from build123d import *

# Parameters (mm, degrees)
F0_R     = 8.5
F1_DEPTH = 18
F3_DEPTH = 11
F4_R     = 10
F5_DEPTH = 11
F7_DEPTH = 10


with BuildPart() as f1:
    # F0 (on Top) → F1 (new body)
    with BuildSketch(Plane.XY):
        Circle(F0_R)
        with BuildLine():
            ThreePointArc((-5.44875, -2.512196), (-5.196152, 3), (-0.54875, 5.974853))
            Line((-0.54875, 5.974853), (5.44875, 2.512196))
            ThreePointArc((5.44875, 2.512196), (5.196152, -3), (0.54875, -5.974853))
            Line((0.54875, -5.974853), (-5.44875, -2.512196))
        make_face(mode=Mode.SUBTRACT)
    extrude(amount=F1_DEPTH)

    # F2 (on Top) → F3 (join)
    with BuildSketch(Plane.XY):
        Polygon((0.509195, 6.881952), (-5.705348, -3.881952), (-0.509195, -6.881952), (0, -6), (5.705348, 3.881952), align=None)
    extrude(amount=F3_DEPTH)

    # F4 (on Top) → F5 (join)
    with BuildSketch(Plane.XY):
        Circle(F4_R)
    extrude(amount=-F5_DEPTH)

    # F6 (on face) → F7 (join)
    with BuildSketch(Plane(origin=(0, 0, -11), x_dir=(1, 0, 0), z_dir=(0, 0, -1))):
        with BuildLine():
            Line((3, -69.539392), (3, -9.539392))
            ThreePointArc((3, -9.539392), (0, 10), (-3, -9.539392))
            Line((-3, -9.539392), (-3, -69.539392))
            Line((-3, -69.539392), (3, -69.539392))
        make_face()
    extrude(amount=F7_DEPTH)


solid = f1.part
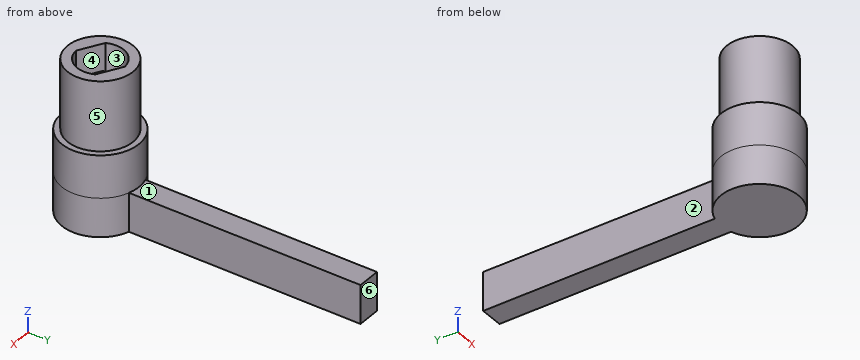
Design review of the part built by this model. Coordinates are the model's own, in mm. Face numbers are marked on the shaded views. A direction names the side the tool comes from. Coordinates: 2 decimals unless noted, no trailing zeros. Loops run counter-clockwise (first coordinate to the right, second up) from the corner with the lowest first, then second, coordinate; pieces in that order, holes last. Notation, with made-up numbers: M 5.25,-5 L 14.25,-5 A22 ccw 14.25,24 Z; hole C 60.25,45 d8. An arc over 180 degrees is marked long. Answer as CSV lines item,"result".
Item 1: The part is to be moulded in two halves that separate along Y. For the marked faces 4, 5 and 6, say which applies: pulls with the +Y half, pulls with the -Y half, needs draft (parallel to the pull), parting line crosses it, or undercut.
Answer list:
face 4,"undercut"
face 5,"parting line crosses it"
face 6,"pulls with the +Y half"
Item 2: Add section C-C on z = -16.5. State the section outline as (x, y) points, plus the area to 3 significant figures.
Answer list:
outline,"M -3,9.54 A10 ccw long 3,9.54 L 3,69.54 L -3,69.54 Z"
area,"672 mm²"
Item 3: For probe 1 along X at (y, z) = (35.5, -15.5); probe 2 along Z at (x, y) = (-2, 29.5); probe 3 along Y at (x, z) = (-5, 11.5), list the stretches that pass through material, from the lowest coordinate up.
Answer list:
probe 1,"-3 to 3"
probe 2,"-21 to -11"
probe 3,"-6.87 to -2.77, 3.32 to 6.87"
Item 4: Machinability: for the marked faces 1, 2 and 3, which of the approach directions +Z, -Z, +X, -X, +Y, -Y give a long, thin tool a straight path to every point of the face, cutting with its end or side? Answer none if there is none.
Answer list:
face 1,"+Z, +X, -X, +Y"
face 2,"+Z, -Z, -X, +Y"
face 3,"+Z"
Item 5: Add section A-A on x = 4.25. State the section outline as (y, z) points.
Answer list:
outline,"M -9.05,-21 L 9.05,-21 L 9.05,0 L 7.36,0 L 7.36,18 L 3.2,18 L 3.2,11 L 1.36,11 L 1.36,0 L -4.24,0 L -4.24,18 L -7.36,18 L -7.36,0 L -9.05,0 Z"
Item 6: Add section D-D on y = 25. State the section outline as (x, z) points.
Answer list:
outline,"M -3,-21 L 3,-21 L 3,-11 L -3,-11 Z"
Item 7: For P1, Ø3, axis at x = 2, y = 0, coming from the +Z side; P2, Ø11, axis at y = 39, z = -14.5, coming from the -X side; P3, Ø4, axis at x = -6.5, z = -4, coming from the +Y side, all flat-tipped, find the tip position at first contact; note any pin that passes through.
Answer list:
P1,"z = 11"
P2,"x = -3"
P3,"y = 8.93"
Item 8: Add section B-B on y = 0. State the section outline as (x, z) points, plus the area to 3 significant figures.
Answer list:
outline,"M -10,-21 L 10,-21 L 10,0 L 8.5,0 L 8.5,18 L 6,18 L 6,0 L 3.46,0 L 3.46,11 L -3.46,11 L -3.46,0 L -6,0 L -6,18 L -8.5,18 L -8.5,0 L -10,0 Z"
area,"586 mm²"
